Could you check a few things on this drawing? It's one solid part, dimensions in mm from its lowest x, y, z. A direction names the side the tool comes from. Give positions to 0.01 mm unless a question says otherwise; leave off trailing zeros. Loops run counter-clockwise (first coordinate to the right, second up) from the corner with the lowest first, then second, coordinate; pieces in that order, holes last. Notation, with made-up numbers: M -20,41.25 L 9,41.25 A16 cw 9,61.25 Z; hole C 79.25,-33.5 d9. An arc over 180 degrees is marked long. Return JSON: item names as keys, results as strings. Group by question number.
1. If we section it at D-D (y = 65): Write out the boundary of the cut face in (x, z) (1 decimal).
2. If we section it at B-B (x = 33.5): Write out the boundary of the cut face in (y, z) (1 decimal).
3. If we section it at C-C (z = 8.5): State how many separate pieces and enclosed holes the cut face has, plus the area to 3 significant figures.
4. If we mould it in two halves opening along X, with no side actions, what happens to the marked faces 1, 2, 3 and 4? For each: +X half, -X half, draft (parallel to the pull), parting line (faces both ways), or undercut.
5. For the marked faces 5 and 6, which set-ups out of +Z, -Z, +X, -X, +Y, -Y let a thin tool reach every point of the face, with its end or its side?
6. For pin 1 (3 mm diameter, centred on x = 45.5, y = 74.5, fed in from -Z); pin 2 (5 mm diameter, centred on x = 75.5, y = 6, fed in from +Z), each with a flat end and sliding along its axis, tell me the tip position at first contact or that it passes through.
7. If we section it at A-A (y = 17): Write out the boundary of the cut face in (x, z) (1 decimal), plus the area to 3 significant figures.
8. Please list where these lines run through material, in increasing order: line 1 (X direction, y = 10.5, z = 8.75) (1 decimal); line 2 (X direction, y = 85, z = 6.25) (1 decimal).
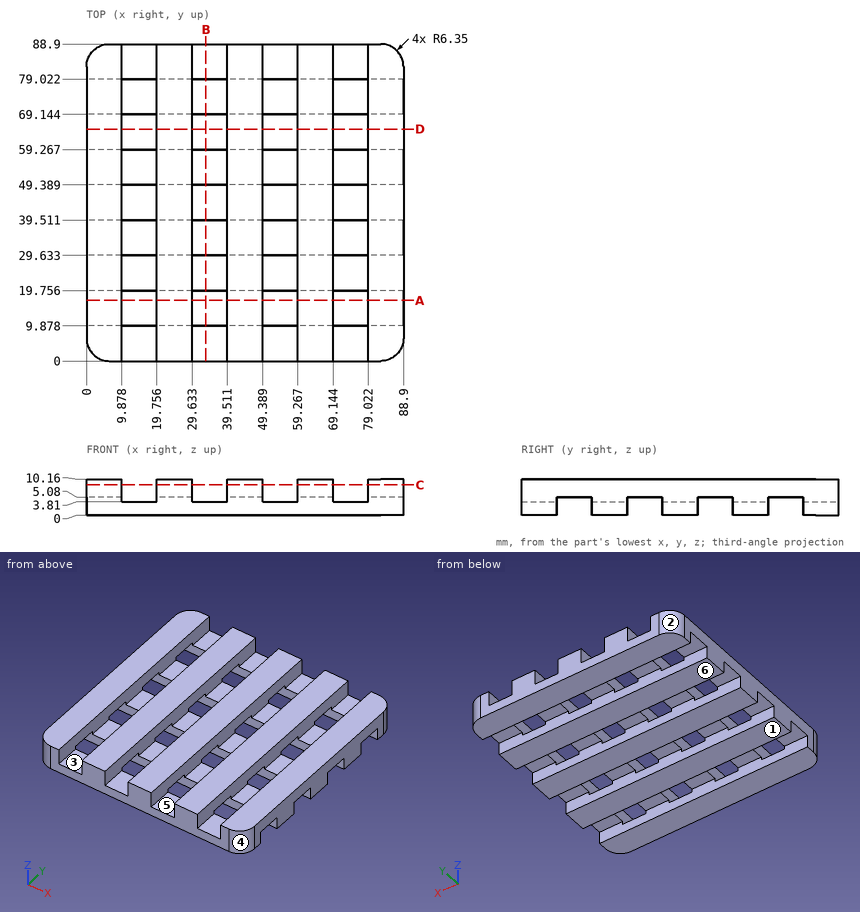
Answer:
{
 "1": {"outline": "M 0,0 L 88.9,0 L 88.9,10.2 L 79,10.2 L 79,3.8 L 69.1,3.8 L 69.1,10.2 L 59.3,10.2 L 59.3,3.8 L 49.4,3.8 L 49.4,10.2 L 39.5,10.2 L 39.5,3.8 L 29.6,3.8 L 29.6,10.2 L 19.8,10.2 L 19.8,3.8 L 9.9,3.8 L 9.9,10.2 L 0,10.2 Z"},
 "2": {"outline": "M 0,0 L 9.9,0 L 9.9,3.8 L 0,3.8 Z; M 19.8,0 L 29.6,0 L 29.6,3.8 L 19.8,3.8 Z; M 39.5,0 L 49.4,0 L 49.4,3.8 L 39.5,3.8 Z; M 59.3,0 L 69.1,0 L 69.1,3.8 L 59.3,3.8 Z; M 79,0 L 88.9,0 L 88.9,3.8 L 79,3.8 Z"},
 "3": {"separate pieces": "5", "enclosed holes": "0", "area": "4,360 mm²"},
 "4": {"face 1": "draft", "face 2": "-X half", "face 3": "undercut", "face 4": "+X half"},
 "5": {"face 5": "+Z, +Y, -Y", "face 6": "-Z, +X, -X, +Y, -Y"},
 "6": {"pin 1": "stops at z = 5.08", "pin 2": "stops at z = 3.81"},
 "7": {"outline": "M 0,5.1 L 9.9,5.1 L 9.9,10.2 L 0,10.2 Z; M 19.8,5.1 L 29.6,5.1 L 29.6,10.2 L 19.8,10.2 Z; M 39.5,5.1 L 49.4,5.1 L 49.4,10.2 L 39.5,10.2 Z; M 59.3,5.1 L 69.1,5.1 L 69.1,10.2 L 59.3,10.2 Z; M 79,5.1 L 88.9,5.1 L 88.9,10.2 L 79,10.2 Z", "area": "251 mm²"},
 "8": {"line 1": "x = 0 to 9.9, 19.8 to 29.6, 39.5 to 49.4, 59.3 to 69.1, 79 to 88.9", "line 2": "x = 0.5 to 9.9, 19.8 to 29.6, 39.5 to 49.4, 59.3 to 69.1, 79 to 88.4"}
}
